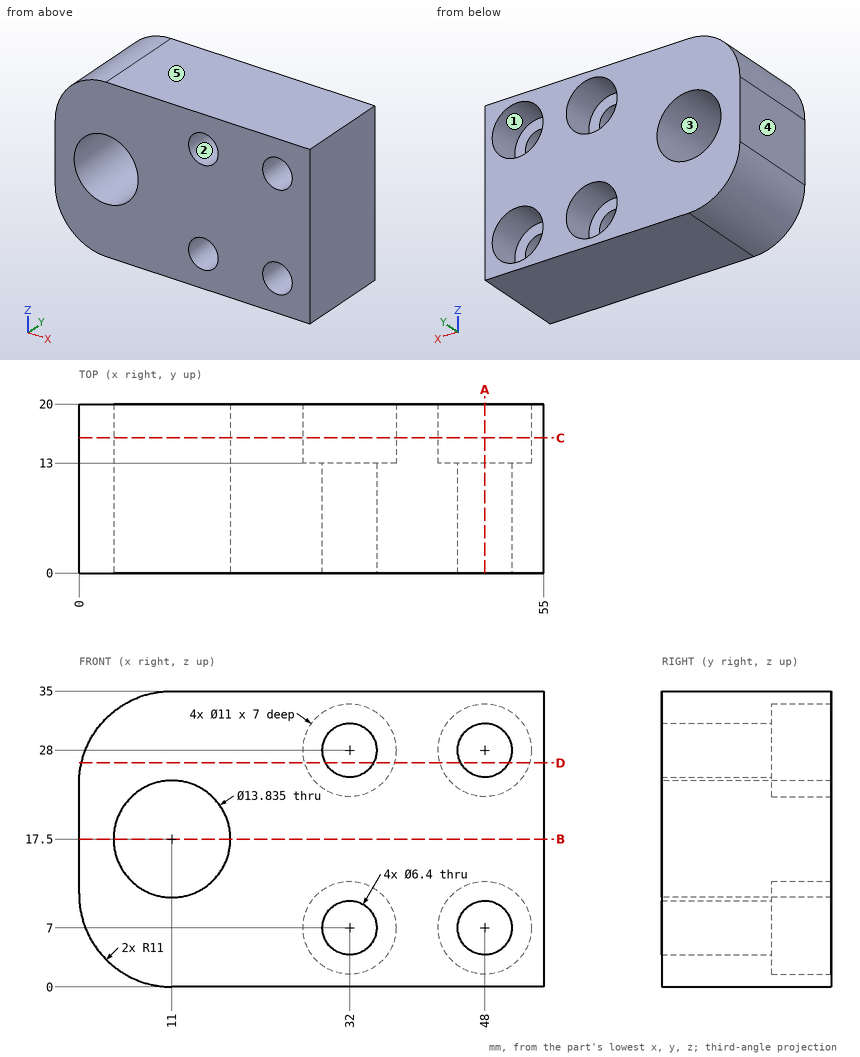
Answer from the drawing. Dimensions are ordinates in mm from the lowest x, y and z of the part. A direction names the side the tool comes from. Coordinates: 2 decimals unless noted, no trailing zeros. Loops run counter-clockwise (first coordinate to the right, second up) from the corner with the lowest first, then second, coordinate; pieces in that order, holes last. Notation, with made-up numbers: (86.25, -25.5) -> (94.25, -25.5) arc R22 cw to (94.25, 13.5) -> close; hole circle Ø3 at (40.5, 3.25). An arc over 180 degrees is marked (long way). Answer in a Markdown table with one row per item.
Item 1: This flat-tipped pin is pushed along its axis until it touches: P1, Ø5.5, axis at x = 30, z = 6.5, coming from the +Y side. Where does it stop, or does it pass through?
Returned:
| item | result |
|---|---|
| P1 | stops at y = 13 |
Item 2: Straight lines are drawn through the part: line 1 along Z through (x, y) = (48, 10); line 2 along Z through (x, y) = (30, 14.5); line 3 along X through (y, z) = (7, 28). For each, find the intervals that lie inside material, in ascending order. Write a range as [from, to].
Returned:
| item | result |
|---|---|
| line 1 | z = [0, 3.8], [10.2, 24.8], [31.2, 35] |
| line 2 | z = [0, 1.88], [12.12, 22.88], [33.12, 35] |
| line 3 | x = [0.75, 28.8], [35.2, 44.8], [51.2, 55] |
Item 3: For a pull along Z with two mould halves and no side action, classify the marked faces 3, 4 and 5 as released by +Z, released by -Z, zero draft, split by the parting line, or undercut.
Returned:
| item | result |
|---|---|
| face 3 | undercut |
| face 4 | zero draft |
| face 5 | released by +Z |
Item 4: A cutting plane is placed at A-A on x = 48. Determine the outline of the cut face in (y, z), plus the area to 3 significant figures.
Returned:
| item | result |
|---|---|
| outline | (0, 0) -> (20, 0) -> (20, 1.5) -> (13, 1.5) -> (13, 3.8) -> (0, 3.8) -> close; (0, 10.2) -> (13, 10.2) -> (13, 12.5) -> (20, 12.5) -> (20, 22.5) -> (13, 22.5) -> (13, 24.8) -> (0, 24.8) -> close; (0, 31.2) -> (13, 31.2) -> (13, 33.5) -> (20, 33.5) -> (20, 35) -> (0, 35) -> close |
| area | 380 mm^2 |
Item 5: A cutting plane is placed at B-B on z = 17.5. Determine the outline of the cut face in (x, y), plus the area to 3 significant figures.
Returned:
| item | result |
|---|---|
| outline | (0, 0) -> (4.08, 0) -> (4.08, 20) -> (0, 20) -> close; (17.92, 0) -> (55, 0) -> (55, 20) -> (17.92, 20) -> close |
| area | 823 mm^2 |
Item 6: For the marked faces 1 and 2, determine the directions among +Z, -Z, +X, -X, +Y, -Y from which every point of the face is accessible in a straight line to the end or side of a thin tool.
Returned:
| item | result |
|---|---|
| face 1 | +Y |
| face 2 | +Y, -Y |
Item 7: A cutting plane is placed at C-C on y = 16. Determine the outline of the cut face in (x, z) (1 decimal).
Returned:
| item | result |
|---|---|
| outline | (0, 11) arc R11 ccw to (11, 0) -> (55, 0) -> (55, 35) -> (11, 35) arc R11 ccw to (0, 24) -> close; hole circle Ø13.8 at (11, 17.5); hole circle Ø11 at (32, 7); hole circle Ø11 at (32, 28); hole circle Ø11 at (48, 7); hole circle Ø11 at (48, 28) |
Item 8: A cutting plane is placed at D-D on z = 26.5. Determine the outline of the cut face in (x, y).
Returned:
| item | result |
|---|---|
| outline | (0.29, 0) -> (29.17, 0) -> (29.17, 13) -> (26.71, 13) -> (26.71, 20) -> (0.29, 20) -> close; (34.83, 0) -> (45.17, 0) -> (45.17, 13) -> (42.71, 13) -> (42.71, 20) -> (37.29, 20) -> (37.29, 13) -> (34.83, 13) -> close; (50.83, 0) -> (55, 0) -> (55, 20) -> (53.29, 20) -> (53.29, 13) -> (50.83, 13) -> close |
